For this review, take the finished solid that the model builds, in its own axes (mm). Coordinates: 2 decimals unless noted, no trailing zeros. Order: outer loops, then holes, each group sorted by start corner. A loop starts at its lowest first (then second) coordinate and runs counter-clockwise, first axis right, second up. Notation, with made-up numbers: (34, 44.5) -> (67, 44.5) arc R14 ccw to (67, 48.5) -> close; hole circle Ø4 at (35, 0.5). An arc over 180 degrees is marked (long way). Answer as a JSON object with one key per item and string values. Group by question number.
1) Add section A-A, the plane x = 30. Write out the cut boundary in (y, z).
2) For pin 1 (9 mm diameter, centred on x = -30, z = 116.35, fed in from -Y); pin 2 (1.5 mm diameter, centred on y = 0.5, z = 138, fed in from +X), all flat-tipped, find the tip position at first contact; note any pin that passes through.
3) Add section B-B, the plane z = 116.35. Write out the cut boundary in (x, y), then the cut area to 3 significant figures.
4) Add section D-D, the plane z = 149. Write out the cut boundary in (x, y).
5) Add section C-C, the plane y = -0.45. Count the separate pieces of the cut face and the enclosed holes in it, then the cut area to 3 significant figures.
6) Wall thickness on L1, parallel to X at y = -0.7, z = 136.35; L2, parallel to X at y = -0.6, z = 76.5; L3, parallel to X at y = 0.8, z = 157: over which ranges is each line inside the solid? List them lowest first.
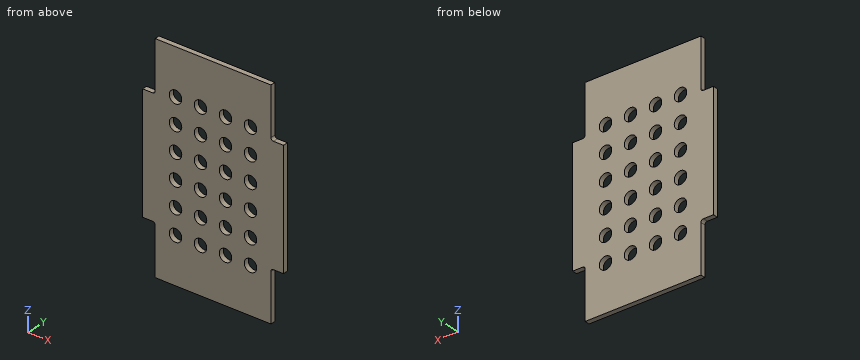
Autodesk Inventor part; units mm, degrees
ref_plane "YZ Plane" through (0, 0, 0) normal (1, 0, 0) x (0, 1, 0)
ref_plane "XZ Plane" through (0, 0, 0) normal (0, 1, 0) x (-1, 0, 0)
ref_plane "XY Plane" through (0, 0, 0) normal (0, 0, 1) x (1, 0, 0)
sketch "Skizze1" plane through (0, 0, 0) normal (0, 0, 1) x (1, 0, 0)
  line L0 (-56.35, 2) -> (56.35, 2)
  line L1 (56.35, 2) -> (56.35, -2)
  line L2 (56.35, -2) -> (-56.35, -2)
  line L3 (-56.35, -2) -> (-56.35, 2)
  line L4 (-56.35, 2) -> (56.35, -2) construction
  line L5 (56.35, 2) -> (-56.35, -2) construction
  point P0 (0, 0)
  dimension "d0" = 4
  dimension "d1" = 112.7
extrude "Extrusion1" add sketch "Skizze1" along normal blind 172.7
sketch "Skizze2" plane through (-56.35, 2, 0) normal (0, 1, 0) x (1, 0, 0)
  circle A0 centre (26.35, -36.35) radius 5
  line L0 (112.7, 0) -> (0, 0)
  line L1 (0, 0) -> (0, -172.7)
  point P0 (56.35, 0)
  dimension "d4" = 10
  dimension "d5" = 36.35
  dimension "d6" = 26.35
extrude "Extrusion2" cut sketch "Skizze2" against normal blind 10
pattern_linear "Rechteckige Anordnung1" count 4 spacing 20 along (1, 0, 0) count 6 spacing 20 along (0, 0, 1) of "Extrusion2"
sketch "Skizze3" plane through (-56.35, 2, 0) normal (0, 1, 0) x (1, 0, 0)
  line L0 (0, -172.7) -> (112.7, -172.7)
  line L1 (0, -172.7) -> (0, -132.7)
  line L2 (0, 0) -> (0, -172.7)
  line L3 (0, -172.7) -> (10, -172.7)
  line L4 (0, 0) -> (112.7, 0)
  line L5 (0, 0) -> (0, -40)
  line L6 (0, 0) -> (10, 0)
  line L7 (112.7, -172.7) -> (102.7, -172.7)
  line L8 (112.7, 0) -> (112.7, -172.7)
  line L9 (112.7, -172.7) -> (112.7, -132.7)
  line L10 (112.7, 0) -> (102.7, 0)
  line L11 (112.7, 0) -> (112.7, -40)
  line L12 (10, -172.7) -> (10, -132.7)
  line L13 (10, -132.7) -> (0, -132.7)
  line L14 (10, 0) -> (10, -40)
  line L15 (10, -40) -> (0, -40)
  circle A0 centre (106.35, -176.35) radius 5
  line L16 (102.7, -172.7) -> (102.7, -132.7)
  line L17 (102.7, -132.7) -> (112.7, -132.7)
  line L18 (102.7, 0) -> (102.7, -40)
  line L19 (102.7, -40) -> (112.7, -40)
  point P0 (56.35, 0)
  point P1 (10, 0)
  point P2 (112.7, -172.9328)
  point P3 (112.7, -179.7672)
  dimension "d15" = 40
  dimension "d17" = 40
  dimension "d19" = 40
  dimension "d20" = 10
  dimension "d21" = 40
  dimension "d22" = 10
  dimension "d25" = 10
  dimension "d26" = 10
extrude "Extrusion3" cut sketch "Skizze3" against normal blind 10 contours L1 L13 L12 L0 | L16 L17 L8 L0 A0 | L2 L4 L14 L15 | A0 L0 | L19 L18 L4 L8 picked at (107.164, -172.1209)
fillet "Rundung1" radius 2 4 edges at (-46.35, 0, 132.7) (-46.35, 0, 40) (46.35, 0, 40) (46.35, 0, 132.7)
properties part number "Schutzglas" material "Glas"
Output values:
{
 "1": {"outline": "(-2, 0) -> (2, 0) -> (2, 31.35) -> (-2, 31.35) -> close; (-2, 41.35) -> (2, 41.35) -> (2, 51.35) -> (-2, 51.35) -> close; (-2, 61.35) -> (2, 61.35) -> (2, 71.35) -> (-2, 71.35) -> close; (-2, 81.35) -> (2, 81.35) -> (2, 91.35) -> (-2, 91.35) -> close; (-2, 101.35) -> (2, 101.35) -> (2, 111.35) -> (-2, 111.35) -> close; (-2, 121.35) -> (2, 121.35) -> (2, 131.35) -> (-2, 131.35) -> close; (-2, 141.35) -> (2, 141.35) -> (2, 172.7) -> (-2, 172.7) -> close"},
 "2": {"pin 1": "passes through", "pin 2": "stops at x = 46.35"},
 "3": {"outline": "(-56.35, -2) -> (-35, -2) -> (-35, 2) -> (-56.35, 2) -> close; (-25, -2) -> (-15, -2) -> (-15, 2) -> (-25, 2) -> close; (-5, -2) -> (5, -2) -> (5, 2) -> (-5, 2) -> close; (15, -2) -> (25, -2) -> (25, 2) -> (15, 2) -> close; (35, -2) -> (56.35, -2) -> (56.35, 2) -> (35, 2) -> close", "area": "291 mm²"},
 "4": {"outline": "(-46.35, -2) -> (46.35, -2) -> (46.35, 2) -> (-46.35, 2) -> close"},
 "5": {"separate pieces": "1", "enclosed holes": "24", "area": "16,000 mm²"},
 "6": {"L1": "x = -46.35 to -35, -25 to -15, -5 to 5, 15 to 25, 35 to 46.35", "L2": "x = -56.35 to -35, -25 to -15, -5 to 5, 15 to 25, 35 to 56.35", "L3": "x = -46.35 to 46.35"}
}
